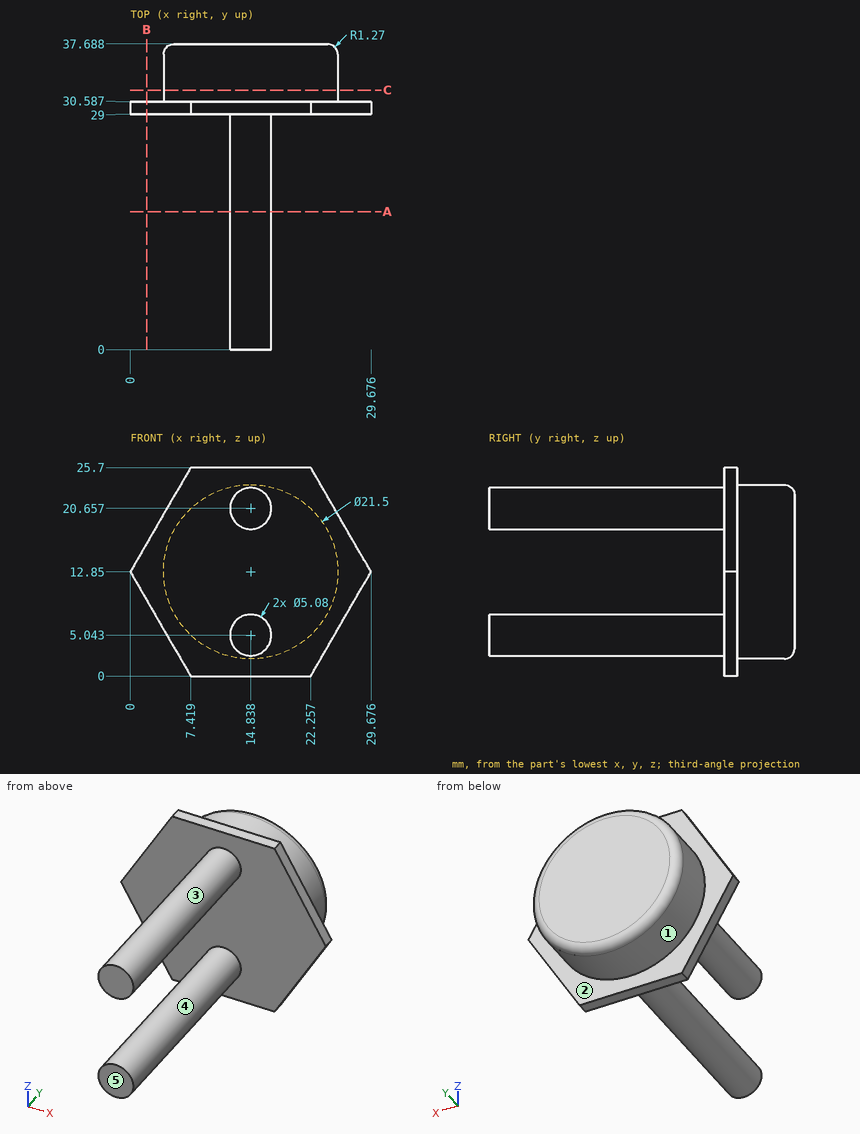
Source: three-view drawing plus pictorial views. Frame: mm from the lowest corner of the part. A direction names the side the tool comes from. Coordinates: 2 decimals unless noted, no trailing zeros. Order: outer loops, then holes, each group sorted by start corner. A loop starts at its lowest first (then second) coordinate and runs counter-clockwise, first axis right, second up.
1) First-contact query: P1, Ø10, axis at x = 11.5, y = 15, coming from the +Z side; P2, Ø4, axis at x = 3.5, z = 8, coming from the -Y side; P3, Ø10, axis at x = 5, y = 12.5, coming from the +Z side; P4, Ø1, axis at x = 7, z = 20.5, coming from the +Y side (1 decimal). Flat tips, straight axial feed; report the tip coordinate or a pass-through.
Result sheet:
P1: stops at z = 23.2
P2: stops at y = 29
P3: passes through
P4: stops at y = 37.2
2) Section A-A (y = 17). Return loops of the section in (x, z).
Result sheet:
outline: circle Ø5.08 at (14.84, 5.04); circle Ø5.08 at (14.84, 20.66)
3) Ray query, probe 1 along Y at (x, z) = (20, 17); probe 2 along Z at (x, y) = (15.5, 23) (1 decimal); probe 3 along Y at (x, z) = (27.5, 15.25). Return the intervals inside material, ascending.
Result sheet:
probe 1: y = 29 to 37.69
probe 2: z = 2.6 to 7.5, 18.2 to 23.1
probe 3: y = 29 to 30.59
4) Section B-B (x = 2). Return loops of the section in (y, z) (1 decimal).
Result sheet:
outline: (29, 9.4) - (30.6, 9.4) - (30.6, 16.3) - (29, 16.3) - close
5) Set-up query: the marked faces 4 and 5. Return all of +Z, -Z, +X, -X, +Y, -Y with unobstructed straight access to the full face (end or side cutting, diameter ignored); none if empty.
Result sheet:
face 4: -Y
face 5: +Z, -Z, +X, -X, -Y
6) Draft query along Z for the marked faces 1, 2 and 3. Return one class per face: released by +Z, released by -Z, zero draft, split by the parting line, or undercut.
Result sheet:
face 1: split by the parting line
face 2: zero draft
face 3: undercut
7) Section C-C (y = 32). Return loops of the section in (x, z).
Result sheet:
outline: circle Ø21.5 at (14.84, 12.85)
